Check sheet for the modelled part. Datum: model origin and axes. Units: mm. Give positions to 0.01 mm unless a question says otherwise; leave off trailing zeros. Loops run counter-clockwise (first coordinate to the right, second up) from the corner with the lowest first, then second, coordinate; pieces in that order, holes last. Notation, with made-up numbers: M 50.25,76 L 71.25,76 A24 cw 71.25,111 Z; hole C 64,39.25 d7. An arc over 180 degrees is marked long. Use one line per item in the form item = value.
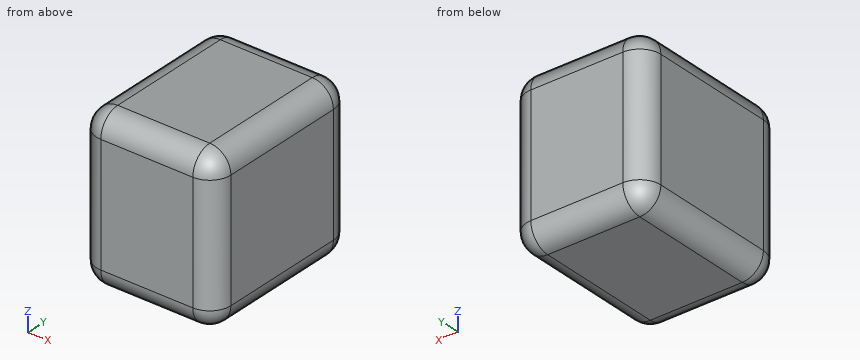
from build123d import *

# Parameters (mm, degrees)
F0_W         = 31.7708179355
F0_H         = 27.5444276631
F1_DEPTH     = 38.1
F2_DEPTH     = 12.7
F3_R         = 5
F4_T1_DEPTH  = 28.1
F4_S5_W      = 5
F4_S5_H      = 5
F4_T6_DEPTH  = 5
F4_S11_W     = 5
F4_S11_H     = 5
F4_T12_DEPTH = 5


# Not quite as in the source:
# - a fillet or chamfer that OpenCascade refuses, or shapes differently, is made with other operations: its cross-section is extruded or revolved along the edge and cut away or added


with BuildPart() as f1:
    # F0 (on Top) → F1 (new body)
    with BuildSketch(Plane.XY):
        with Locations((15.8854089677, -13.7722138315)):
            Rectangle(F0_W, F0_H)
    extrude(amount=F1_DEPTH)

    # F2 (add): a face of the model
    f2_faces = [f1.faces().sort_by_distance(p)[0] for p in [
        (15.8854089677, -27.5444276631, 19.05),
    ]]
    extrude(f2_faces, amount=F2_DEPTH)

    # F3
    f3_edges = [f1.edges().sort_by_distance(p)[0] for p in [
        (0, -40.244428, 19.05),
        (0, -20.122214, 38.1),
        (31.770818, -20.122214, 0),
        (31.770818, -20.122214, 38.1),
        (31.770818, -40.244428, 19.05),
        (15.885409, 0, 38.1),
        (15.885409, -40.244428, 0),
        (0, -20.122214, 0),
        (15.885409, -40.244428, 38.1),
        (15.885409, 0, 0),
        (0, 0, 19.05),
    ]]
    fillet(f3_edges, radius=F3_R)

    # F4: fillet of radius 5 on 1 edges, made by hand

    # F4_s2 → F4_t1 (cut)
    with BuildSketch(Plane.XY.offset(5)):
        with BuildLine():
            ThreePointArc((26.7708179355, 0), (30.3063518414, -1.4644660941), (31.7708179355, -5))
            Line((31.7708179355, -5), (31.7708179355, 0))
            Line((31.7708179355, 0), (26.7708179355, 0))
        make_face()
    extrude(amount=F4_T1_DEPTH, mode=Mode.SUBTRACT)


with BuildPart() as f4_tool4:
    # F4_s5 → F4_t6 (new body)
    with BuildSketch(Plane.XZ.offset(5)):
        with Locations((29.2708179355, 2.5)):
            Rectangle(F4_S5_W, F4_S5_H)
    extrude(amount=-F4_T6_DEPTH)

    # F4_s7 → F4_t8 (revolve, cut)
    with BuildSketch(Plane(origin=(26.7708179355, -5, 5), x_dir=(-0.7071067812, 0, 0.7071067812), z_dir=(-0.7071067812, 0, -0.7071067812))):
        with BuildLine():
            ThreePointArc((0, -5), (5, 0), (0, 5))
            Line((0, 5), (0, -5))
        make_face()
    revolve(axis=Axis((26.7708179355, -5, 5), (0, 1, 0)), mode=Mode.SUBTRACT)


with BuildPart() as f1_1:
    add(f1.part)

    # F4_t3: cut F4_tool4
    add(f4_tool4.part, mode=Mode.SUBTRACT)


with BuildPart() as f4_tool10:
    # F4_s11 → F4_t12 (new body)
    with BuildSketch(Plane.XZ.offset(5)):
        with Locations((29.2708179355, 35.6)):
            Rectangle(F4_S11_W, F4_S11_H)
    extrude(amount=-F4_T12_DEPTH)

    # F4_s13 → F4_t14 (revolve, cut)
    with BuildSketch(Plane(origin=(26.7708179355, -5, 33.1), x_dir=(-0.7071067812, 0, -0.7071067812), z_dir=(0.7071067812, 0, -0.7071067812))):
        with BuildLine():
            ThreePointArc((0, -5), (5, 0), (0, 5))
            Line((0, 5), (0, -5))
        make_face()
    revolve(axis=Axis((26.7708179355, -5, 33.1), (0, 1, 0)), mode=Mode.SUBTRACT)


with BuildPart() as f1_2:
    add(f1_1.part)

    # F4_t9: cut F4_tool10
    add(f4_tool10.part, mode=Mode.SUBTRACT)


solid = f1_2.part
1) Depth check by flat-ended pin: pin 1 Ø1.5 at (x, z) = (28, 9) entering from -Y. Enter the tip coordinate at first touch or a pass-through.
Evaluation:
pin_1 = -40.22
2) Section check B-B (y = -33). Record the cut outline in (x, z), then the cut area to 3 significant figures.
Evaluation:
outline = M 0,5 A5 ccw 5,0 L 26.77,0 A5 ccw 31.77,5 L 31.77,33.1 A5 ccw 26.77,38.1 L 5,38.1 A5 ccw 0,33.1 Z
area = 1,190 mm^2
3) Section check A-A (z = 30.5). Record the cut outline in (x, y).
Evaluation:
outline = M 0,-35.24 A5 ccw 5,-40.24 L 26.77,-40.24 A5 ccw 31.77,-35.24 L 31.77,-5 A5 ccw 26.77,0 L 5,0 A5 ccw 0,-5 Z
4) Scan lines: line 1 (Z direction, x = 27, y = -20); line 2 (Z direction, x = 15, y = -37); line 3 (Y direction, x = 27, z = 14). Record each from-to range of solid material in increasing order.
Evaluation:
line_1 = 0.01 to 38.09
line_2 = 0.32 to 37.78
line_3 = -40.24 to -0.01
